Autodesk Inventor part; units mm, degrees
ref_plane "YZ Plane" through (0, 0, 0) normal (1, 0, 0) x (0, 1, 0)
ref_plane "XZ Plane" through (0, 0, 0) normal (0, 1, 0) x (-1, 0, 0)
ref_plane "XY Plane" through (0, 0, 0) normal (0, 0, 1) x (1, 0, 0)
sketch "Sketch1" plane through (0, 0, 0) normal (0, 1, 0) x (-1, 0, 0)
  line L0 (0, 0) -> (-12.7, 0)
  line L1 (-12.7, 0) -> (-12.7, -25.4)
  line L2 (-12.7, -25.4) -> (0, -25.4)
  line L3 (0, -25.4) -> (0, 0)
  line L4 (-2.54, -2.54) -> (-10.16, -2.54)
  line L5 (-10.16, -2.54) -> (-10.16, -6.0325)
  line L6 (-10.16, -6.0325) -> (-2.54, -6.0325)
  line L7 (-2.54, -6.0325) -> (-2.54, -2.54)
  circle A0 centre (-3.175, -8.5725) radius 0.635
  circle A1 centre (-9.525, -8.5725) radius 0.635
  line L8 (-2.54, -19.3675) -> (-10.16, -19.3675)
  line L9 (-10.16, -19.3675) -> (-10.16, -22.86)
  line L10 (-10.16, -22.86) -> (-2.54, -22.86)
  line L11 (-2.54, -22.86) -> (-2.54, -19.3675)
  dimension "d0" = 12.7
  dimension "d1" = 25.4
  dimension "d2" = 2.54
  dimension "d3" = 2.54
  dimension "d4" = 2.54
  dimension "d5" = 1.27
  dimension "d6" = 2.54
  dimension "d7" = 2.54
  dimension "d8" = 2.54
extrude "Extrusion1" add sketch "Sketch1" along normal blind 12.7
extrude "Extrusion2" add sketch "Sketch1" along normal blind 0.508 contours L7 L6 L5 L4 | A0 | A1 | L11 L10 L9 L8
properties part number "Wrist Base"
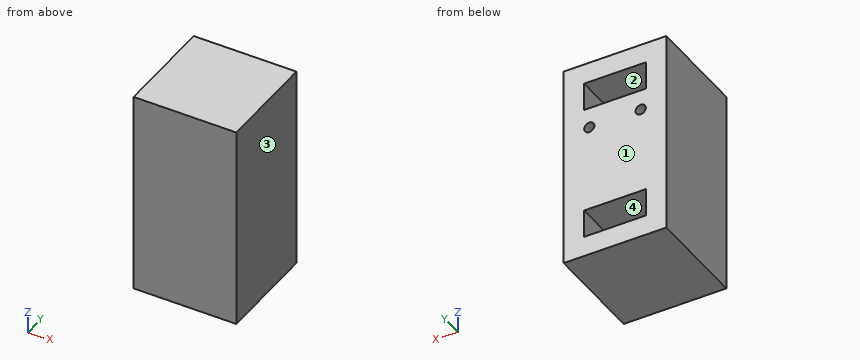
Source: CAD feature listing. Evaluate the final solid. Frame: model axes, mm. Face numbers are marked on the shaded views. Coordinates: 2 decimals unless noted, no trailing zeros. Loops run counter-clockwise (first coordinate to the right, second up) from the corner with the lowest first, then second, coordinate; pieces in that order, holes last. Notation, with made-up numbers: M 88,-3 L 94,-3 A16 cw 94,6 Z; hole C -3.75,70.25 d8. An arc over 180 degrees is marked long. Use a Markdown table: item, result. Add a question column.
Q1. Draft query along X for the marked faces 1, 2, 3 and 4. Return one class per face: pulls with the +X half, pulls with the -X half, needs draft (parallel to the pull), parting line crosses it, or undercut.
Q2. Material intervals for L1, parallel to Z at x = 5, y = 5.75; L2, parallel to Z at x = 3.25, y = 6.5; L3, parallel to X at y = 1.5, z = -8.5, sorted ascending.
Q3. Section query B-B, the plane x = 4.75. Return loops of the section in (y, z).
Q4. Section query A-A, the plane z = -3.75. Return loops of the section in (x, y).
Q5. Section query C-C, the plane y = 9. Return loops of the section in (x, z) (1 decimal).
Q6. First-contact query: pin 1 (3 mm diameter, centred on x = 6.5, z = -4.5, fed in from +Y); pin 2 (1.5 mm diameter, centred on y = 1.5, z = -10, fed in from -X). Flat tips, straight axial feed; report the tip coordinate or a pass-through.
Result:
| question | item | result |
|---|---|---|
| 1 | face 1 | needs draft |
| 1 | face 2 | undercut |
| 1 | face 3 | pulls with the +X half |
| 1 | face 4 | undercut |
| 2 | L1 | z = -25.4 to -22.86, -19.37 to -6.03, -2.54 to 0 |
| 2 | L2 | z = -25.4 to -22.86, -19.37 to -9.2, -7.94 to -6.03, -2.54 to 0 |
| 2 | L3 | x = 0 to 2.54, 3.81 to 8.89, 10.16 to 12.7 |
| 3 | outline | M 0,-25.4 L 12.7,-25.4 L 12.7,-22.86 L 0.51,-22.86 L 0.51,-19.37 L 12.7,-19.37 L 12.7,-6.03 L 0.51,-6.03 L 0.51,-2.54 L 12.7,-2.54 L 12.7,0 L 0,0 Z |
| 4 | outline | M 0,0 L 12.7,0 L 12.7,12.7 L 10.16,12.7 L 10.16,0.51 L 2.54,0.51 L 2.54,12.7 L 0,12.7 Z |
| 5 | outline | M 0,-25.4 L 12.7,-25.4 L 12.7,0 L 0,0 Z; hole M 2.5,-22.9 L 10.2,-22.9 L 10.2,-19.4 L 2.5,-19.4 Z; hole C 3.2,-8.6 d1.3; hole M 2.5,-6 L 10.2,-6 L 10.2,-2.5 L 2.5,-2.5 Z; hole C 9.5,-8.6 d1.3 |
| 6 | pin 1 | stops at y = 0.51 |
| 6 | pin 2 | stops at x = 0 |
